CAD build for the part. Positions are in the model's coordinates, mm. Face numbers are marked on the shaded views. A direction names the side the tool comes from. Give positions to 0.01 mm unless a question says otherwise; leave off trailing zeros. Write each loop counter-clockwise with the first axis right and the second up, starting at its lowest first coordinate (ties: lowest second). Pieces come first, ordered by that corner, then holes. Notation, with made-up numbers: (52, 71) -> (105, 71) arc R17 cw to (105, 96) -> close; hole circle Ø3 at (87.25, 88.5). An arc over 180 degrees is marked (long way). Answer as a JSON object with one key per item and string values.
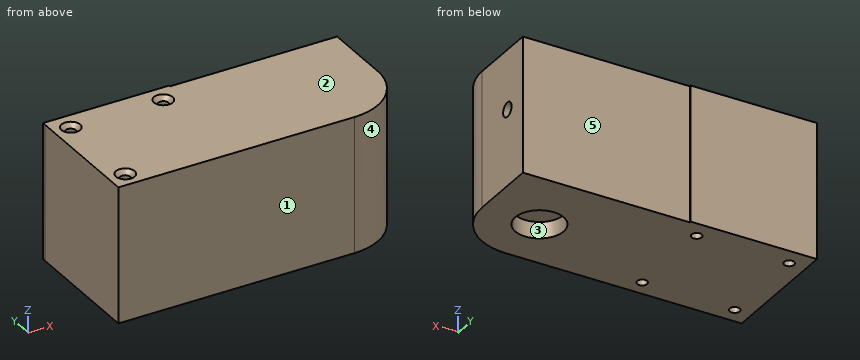
Autodesk Inventor part; units mm, degrees
ref_plane "Work Plane1" through (-349.1377, -7.0016, 45.5) normal (0, 0, 1) x (1, -0.0015, 0)
ref_plane "YZ Plane" through (0, 0, 0) normal (1, 0, 0) x (0, 1, 0)
ref_plane "XZ Plane" through (0, 0, 0) normal (0, 1, 0) x (-1, 0, 0)
sketch "Sketch1" plane through (0, 0, 0) normal (0, 0, 1) x (1, 0, 0)
  arc A0 (14.1427, -15.2387) -> (13.4175, -14.0632) centre (13.1646, -15.0307) ccw
  line L0 (13.4175, -14.0632) -> (9.4746, -13.0327)
  arc A1 (9.4746, -13.0327) -> (0.5427, -12.0878) centre (1.8884, -42.0576) ccw
  arc A2 (1.3475, 12.0247) -> (0.5427, -12.0878) centre (0, 0) ccw
  arc A3 (1.3475, 12.0247) -> (10.3225, 12.3719) centre (4.6883, 41.8381) ccw
  line L1 (10.3225, 12.3719) -> (21.175, 14.447)
  line L2 (21.175, 14.447) -> (21.175, 21.6191)
  line L3 (-21.175, 20.6809) -> (-21.175, -21.125)
  line L4 (-21.175, -21.125) -> (21.175, -21.125)
  line L5 (21.175, -21.125) -> (21.175, -16.0908)
  line L6 (21.175, -16.0908) -> (17.9879, -15.2578)
  arc A4 (17.9879, -15.2578) -> (16.7802, -15.9281) centre (17.735, -16.2253) ccw
  arc A5 (14.1427, -15.2387) -> (16.7802, -15.9281) centre (15.4774, -15.5226) ccw
  circle A6 centre (-15.4774, 15.5226) radius 1.3645
  circle A7 centre (-15.5226, -15.4774) radius 1.3645
  circle A8 centre (15.5226, 15.4774) radius 1.3645
  circle A9 centre (57.9677, -1.9346) radius 4.2
  circle A10 centre (57.9677, -1.9346) radius 19.1904
  line L7 (21.175, -21.125) -> (57.9677, -21.125)
  line L8 (21.175, 21.125) -> (77.1581, 21.125)
  line L9 (77.1581, 21.125) -> (77.1581, -1.9346)
  line L10 (-21.1741, 21.6809) -> (21.175, 21.6191)
  line L11 (-21.1741, 21.6809) -> (-21.1756, 20.6809)
  line L12 (-21.175, 20.6809) -> (-21.1756, 20.6809)
  point P0 (0, 0)
  point P1 (-21.175, 21.125)
extrude "Extrusion1" add sketch "Sketch1" along normal blind 5.5
sketch "Sketch2" plane through (0, 0, 5.5) normal (0, 0, 1) x (1, 0, 0)
  line L0 (77.1581, -1.9346) -> (77.1581, 21.125)
  line L1 (-21.175, 20.6809) -> (-21.175, -21.125)
  line L2 (-21.175, -21.125) -> (57.9677, -21.125)
  arc A0 (57.9677, -21.125) -> (77.1581, -1.9346) centre (57.9677, -1.9346) ccw
  circle A1 centre (15.5226, 15.4774) radius 1.3645
  circle A2 centre (-15.5226, -15.4774) radius 1.3645
  circle A3 centre (-15.4774, 15.5226) radius 1.3645
  circle A4 centre (57.9677, -1.9346) radius 4.2
  line L3 (110.8694, -1.8119) -> (-349.1301, -1.1403)
  line L4 (110.8699, -1.5119) -> (-349.1296, -0.8403)
  line L5 (21.175, 21.6191) -> (-21.1741, 21.6809)
  line L6 (-21.1741, 21.6809) -> (-21.1756, 20.6809)
  line L7 (-21.1756, 20.6809) -> (-21.175, 20.6809)
  line L8 (77.1581, 21.125) -> (21.175, 21.125)
  line L9 (21.175, 21.125) -> (21.175, 21.6191)
  point P0 (0, 0)
  point P1 (-21.175, -1.3191)
  point P2 (77.1581, -1.4626)
  dimension "d2" = 0.3
ref_plane "Work Plane1" through (-349.1377, -7.0016, 45.5) normal (0, 0, 1) x (1, -0.0015, 0)
extrude "Extrusion2" add sketch "Sketch2" along normal up to surface (40 mm away) contours A0 L2 L1 L3 A4 L0 | L3 A4 L4 L0 | L4 A4 L1 L6 L5 L9 L8 L0 | L3 A4 L4 | A4 L3 | L4 A4 | L3 L1 L4 A4 | A2
sketch "Sketch3" plane through (-21.175, 26.125, 0) normal (0, 1, 0) x (1, 0, 0)
  line L0 (-327.9643, -38.4057) -> (-327.9643, -32.5943)
  line L1 (132.0352, -38.4057) -> (-327.9643, -38.4057)
  line L2 (132.0352, -38.4057) -> (132.0352, -32.5943)
  line L3 (132.0352, -32.5943) -> (-327.9643, -32.5943)
  line L4 (-327.9643, -18.4057) -> (-327.9643, -12.5943)
  line L5 (132.0352, -18.4057) -> (-327.9643, -18.4057)
  line L6 (132.0352, -18.4057) -> (132.0352, -12.5943)
  line L7 (132.0352, -12.5943) -> (-327.9643, -12.5943)
  line L8 (98.3331, 0) -> (98.3331, -45.5)
  line L9 (0, 0) -> (0, -45.5)
  point P0 (21.175, 0)
  point P1 (83.3331, -35.5)
  point P2 (83.3331, -35.5)
  point P3 (15, -15.5)
  point P4 (83.3331, -15.5)
  point P5 (15, -35.5)
  dimension "d8" = 15
  dimension "d9" = 15
hole "Hole1" [suppressed]
sketch "Sketch4" plane through (-21.175, 26.125, 45.5) normal (0, 0, 1) x (1, 0, 0)
  circle A0 centre (36.6976, -10.6476) radius 1.3645
  circle A1 centre (5.6976, -10.6024) radius 1.3645
  circle A2 centre (5.6523, -41.6024) radius 1.3645
  point P0 (21.175, -26.125)
hole "Hole2" at (15.5226, 15.4774, 45.5) at (-15.4774, 15.5226, 45.5) at (-15.5226, -15.4774, 45.5) direction (0, 0, -1) diameter 3.4 end through all countersink diameter 6.3 countersink angle 90
sketch "Sketch5" plane through (0, 0, 0) normal (0, 0, -1) x (-1, 0, 0)
  arc A0 (-62.1677, -1.9346) -> (-62.1677, -1.9346) centre (-57.9677, -1.9346) ccw
  circle A1 centre (-57.9677, -1.9346) radius 8.1
  point P0 (0, 0)
  dimension "d24" = 16.2
extrude "Extrusion3" cut sketch "Sketch5" against normal up to surface (5.5 mm away) contours A0 | A1
sketch "Sketch6" plane through (0, 0, 5.5) normal (0, 0, 1) x (1, 0, 0)
  circle A0 centre (15.4774, -15.5226) radius 2.3806
  circle A1 centre (-15.5226, -15.4774) radius 1.7
  point P0 (0, 0)
hole "Hole3" at (15.4774, -15.5226, 5.5) at (-15.5226, -15.4774, 5.5) direction (0, 0, -1) diameter 3.4 end through all countersink diameter 6.3 countersink angle 90
sketch "Sketch7" plane through (77.1581, -1.9346, 5.5) normal (1, 0, 0) x (0, 0, -1)
  circle A0 centre (-20, 14.2658) radius 4.5
  point P0 (5.5, 1.9346)
hole "Hole4" at (77.1581, 12.3312, 25.5) direction (-1, 0, 0) diameter 4.8 depth 20
properties part number "PRINTED right z mount 2"
1) Slice it at D-D (z = 7.5). List the corners of the cut face in (x, y) (3 decimals), then the cut area to 3 significant figures.
Model answer:
{"outline": "(-21.175, -21.125) -> (57.968, -21.125) arc R19.19 ccw to (77.158, -1.935) -> (77.158, 21.125) -> (21.175, 21.125) -> (21.175, 21.619) -> (-21.174, 21.681) -> (-21.175, 20.681) -> close; hole circle Ø3.4 at (-15.523, -15.477); hole circle Ø3.4 at (-15.477, 15.523); hole circle Ø3.4 at (15.523, 15.477)", "area": "4,070 mm2"}
2) Wall check: probe 1 along X at (y, z) = (14.5, 6.5) (3 decimals); probe 2 along X at (y, z) = (15, 5.5) (3 decimals); probe 3 along Y at (x, z) = (69, 25) (3 decimals). Give the ranges that are in metal, low to high.
Model answer:
{"probe 1": "x = -21.175 to -16.835, -14.119 to 14.132, 16.914 to 77.158", "probe 2": "x = -21.175 to -17.095, -13.86 to 13.891, 17.154 to 77.158", "probe 3": "y = -17.637 to 9.984, 14.679 to 21.125"}
3) Slice it at B-B (z = 25.5). List the corners of the cut face in (x, y) (3 decimals).
Model answer:
{"outline": "(-21.175, -21.125) -> (57.968, -21.125) arc R19.19 ccw to (77.158, -1.935) -> (77.158, 9.931) -> (57.158, 9.931) -> (57.158, 14.731) -> (77.158, 14.731) -> (77.158, 21.125) -> (21.175, 21.125) -> (21.175, 21.619) -> (-21.174, 21.681) -> (-21.175, 20.681) -> close; hole circle Ø3.4 at (-15.523, -15.477); hole circle Ø3.4 at (-15.477, 15.523); hole circle Ø3.4 at (15.523, 15.477)"}
4) Slice it at A-A (x = 59.5). List the corners of the cut face in (y, z) (3 decimals), then the cut area to 3 significant figures.
Model answer:
{"outline": "(-21.064, 0) -> (-9.888, 0) -> (-9.888, 5.5) -> (6.019, 5.5) -> (6.019, 0) -> (21.125, 0) -> (21.125, 45.5) -> (-21.064, 45.5) -> close; hole circle Ø4.8 at (12.331, 25.5)", "area": "1,810 mm2"}
5) Mould opens along Y. For the marked faces 1, 2 and 3 say: released by +Y, released by -Y, zero draft, split by the parting line, or undercut.
Model answer:
{"face 1": "released by -Y", "face 2": "zero draft", "face 3": "undercut"}
6) Slice it at C-C (y = 1). List the corners of the cut face in (x, z) (3 decimals).
Model answer:
{"outline": "(-21.175, 0) -> (50.418, 0) -> (50.418, 5.5) -> (65.517, 5.5) -> (65.517, 0) -> (77.158, 0) -> (77.158, 45.5) -> (-21.175, 45.5) -> close"}
7) 3-axis set-ups, long thin cutter, end or side, ignore diameter. For the marked faces 4 and 5: which of +Z, -Z, +X, -X, +Y, -Y reach the whole face in a straight line?
Model answer:
{"face 4": "+Z, -Z, +X, -Y", "face 5": "+Z, -Z, +X, +Y"}
8) Pin check, flat tips, straight feed: pin 1 (5.5 mm diameter, centred on x = 15.52, y = 15.48, fed in from +Z); pin 2 (2.5 mm diameter, centred on y = 12.5, z = 26, fed in from +X); pin 3 (0.5 mm diameter, centred on y = 21.5, z = 20.5, fed in from +X) (3 decimals). Stop position of each tip, or through.
Model answer:
{"pin 1": "stops at z = 45.1", "pin 2": "stops at x = 57.16", "pin 3": "stops at x = 21.175"}
